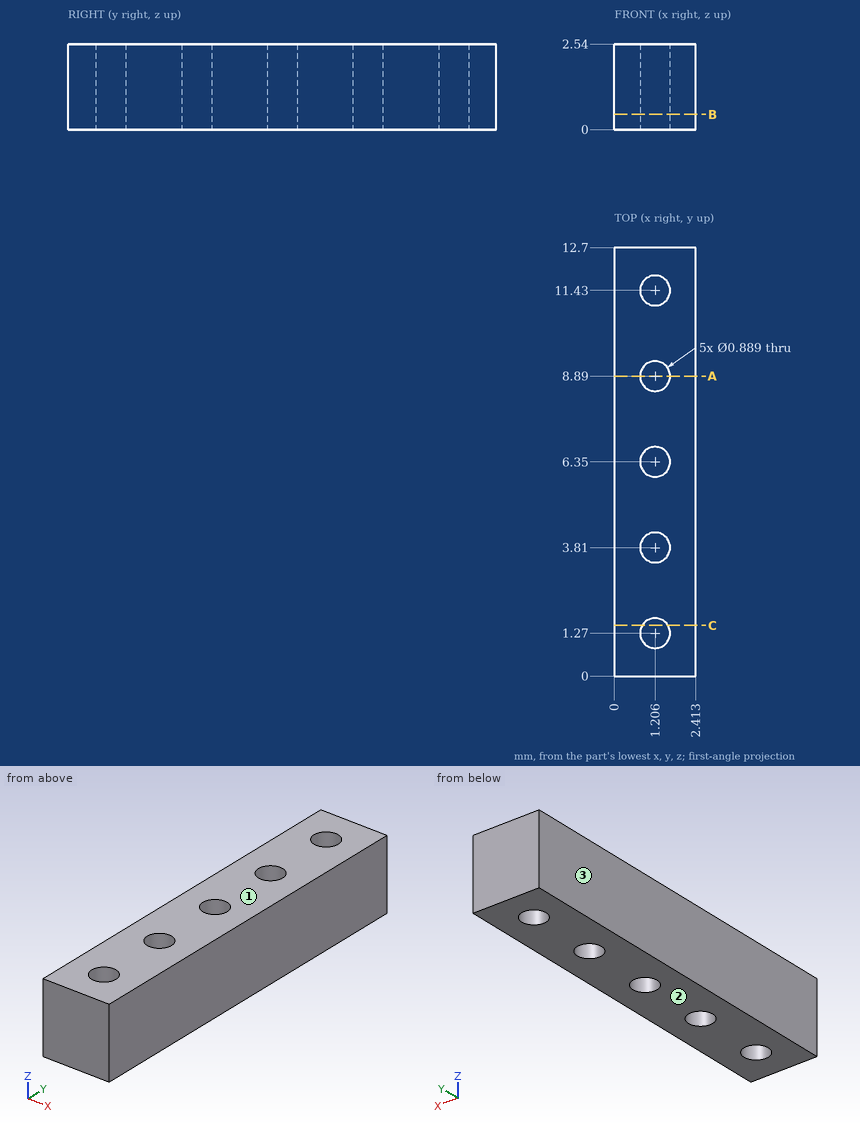
Geometry check sheet. Reference: drawing and pictorial views, mm from the part's lowest x, y, z. Coordinates: 2 decimals unless noted, no trailing zeros. Order: outer loops, then holes, each group sorted by start corner. A loop starts at its lowest first (then second) coordinate and runs counter-clockwise, first axis right, second up.
Item 1: Mould release check, pull along Z, two halves, no side actions. Record for the marked faces 1, 2 and 3: released by +Z, released by -Z, zero draft, split by the parting line, or undercut.
Item 2: Section check B-B (z = 0.45). Count the separate pieces of the cut face and the enclosed holes in it.
Item 3: Depth check by flat-ended pin: pin 1 (1 mm diameter, centred on x = 0.5, y = 4, fed in from -Z). Enter the tip coordinate at first touch or a pass-through.
Item 4: Section check A-A (y = 8.89). Enter the section's corners in (x, z).
Item 5: Scan lines: line 1 along Y through (x, z) = (1.1, 2.45); line 2 along X through (y, z) = (6.5, 0.4) (1 decimal). Record each from-to range of solid material in increasing order.
Item 6: Section check C-C (y = 1.5). Enter the section's corners in (x, z).
Check sheet entries:
1. face 1: released by +Z
1. face 2: released by -Z
1. face 3: zero draft
2. separate pieces: 1
2. enclosed holes: 5
3. pin 1: stops at z = 0
4. outline: (0, 0) - (0.76, 0) - (0.76, 2.54) - (0, 2.54) - close; (1.65, 0) - (2.41, 0) - (2.41, 2.54) - (1.65, 2.54) - close
5. line 1: y = 0 to 0.84, 1.7 to 3.38, 4.24 to 5.92, 6.78 to 8.46, 9.32 to 11, 11.86 to 12.7
5. line 2: x = 0 to 0.8, 1.6 to 2.4
6. outline: (0, 0) - (0.83, 0) - (0.83, 2.54) - (0, 2.54) - close; (1.59, 0) - (2.41, 0) - (2.41, 2.54) - (1.59, 2.54) - close
